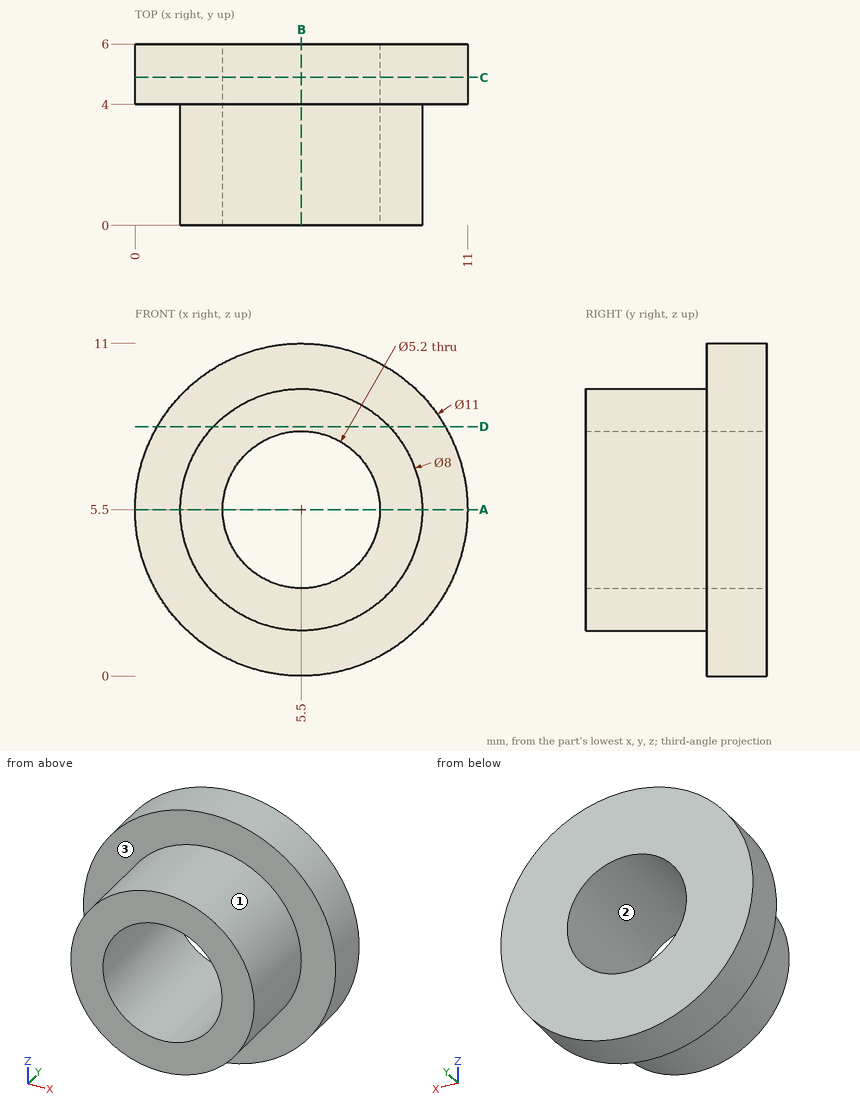
For this review, use the dimensioned drawing (mm, ordinates from the lowest corner) and the shaded views. Coordinates: 2 decimals unless noted, no trailing zeros. Write each loop counter-clockwise with the first axis right and the second up, starting at its lowest first coordinate (ties: lowest second). Pieces come first, ordered by that corner, then holes. Notation, with made-up numbers: (42, 16) - (77, 16) arc R17 ccw to (77, 34) - close; hole circle Ø3 at (45.25, 45). An arc over 180 degrees is marked (long way). Answer in a Markdown table with one row per item. Add a question column.
Q1. Consider section A-A on z = 5.5. Give the boundary of the cut face in (x, y).
Q2. Consider section D-D on z = 8.25. Give the boundary of the cut face in (x, y), then the cut area to 3 significant figures.
Q3. Draft analysis for pull direction X (two halves, no side actions). For the marked faces 1, 2 and 3, state which applies: +X half, -X half, draft (parallel to the pull), parting line (faces both ways), or undercut.
Q4. To check wall thickness, follow line 1 along Z through (x, y) = (5.5, 3.4); line 2 along Z through (x, y) = (5.5, 4.45). State the ranges of each line that lie inside material, in increasing order. Write a range as from..to.
Q5. Consider section C-C on y = 4.9. Give the boundary of the cut face in (x, z), then the cut area to 3 significant figures.
Q6. Clearance check with flat-ended pins moving along their axes: pin 1 (1.5 mm diameter, centred on x = 6.5, y = 2, fed in from -Z); pin 2 (1 mm diameter, centred on x = 6, z = 5, fed in from +Y); pin 3 (1.5 mm diameter, centred on y = 3.5, z = 9.5, fed in from +X). State where each tip first meets the part, or that it passes through.
Q7. Consider section B-B on x = 5.5. Give the boundary of the cut face in (y, z), then the cut area to 3 significant figures.
Answers below:
| question | item | result |
|---|---|---|
| 1 | outline | (0, 4) - (1.5, 4) - (1.5, 0) - (2.9, 0) - (2.9, 6) - (0, 6) - close; (8.1, 0) - (9.5, 0) - (9.5, 4) - (11, 4) - (11, 6) - (8.1, 6) - close |
| 2 | outline | (0.74, 4) - (2.6, 4) - (2.6, 0) - (8.4, 0) - (8.4, 4) - (10.26, 4) - (10.26, 6) - (0.74, 6) - close |
| 2 | area | 42.3 mm² |
| 3 | face 1 | parting line |
| 3 | face 2 | undercut |
| 3 | face 3 | draft |
| 4 | line 1 | 1.5..2.9, 8.1..9.5 |
| 4 | line 2 | 0..2.9, 8.1..11 |
| 5 | outline | circle Ø11 at (5.5, 5.5); hole circle Ø5.2 at (5.5, 5.5) |
| 5 | area | 73.8 mm² |
| 6 | pin 1 | z = 1.51 |
| 6 | pin 2 | through |
| 6 | pin 3 | x = 9.79 |
| 7 | outline | (0, 1.5) - (4, 1.5) - (4, 0) - (6, 0) - (6, 2.9) - (0, 2.9) - close; (0, 8.1) - (6, 8.1) - (6, 11) - (4, 11) - (4, 9.5) - (0, 9.5) - close |
| 7 | area | 22.8 mm² |
